Source: CAD feature listing. Evaluate the final solid. Frame: model axes, mm. A direction names the side the tool comes from. Coordinates: 2 decimals unless noted, no trailing zeros. Write each loop counter-clockwise with the first axis right and the second up, starting at its lowest first coordinate (ties: lowest second). Pieces come first, ordered by that corner, then holes. Notation, with made-up numbers: (86, -26.5) - (137, -26.5) arc R9 ccw to (137, -14.5) - close; hole circle Ø5 at (-13.75, -36). An arc over 180 degrees is marked (long way). One line per question, with ' | ' between items. Start each with the question number.
Q1. Draft query along Y for faces 1 (the face through (15, -9, 2)), 2 (the face through (-1.301, 19.143, 2.958)), 3 (the face through (14.43, -26.6, 7.04)), 4 (the face through (-12.341, -18.443, 6.958)). Return one class per face: +Y half, -Y half, draft (parallel to the pull), parting line (faces both ways), or undercut.
Q2. Contact query for flat-ended pins moving along their axis: P1, Ø1, axis at x = 11, y = -10, coming from the +Z side; P2, Ø17.5, axis at x = 2, y = 23.5, coming from the +Z side; P3, Ø3, axis at x = 2.5, z = 6, coming from the +Y side. Output: stop coordinate, or through.
Q3. Cut plane A-A, the plane y = 25. Return loops of the section in (x, z).
Q4. Access query for faces 5 (the face through (2, -26, 7)), 6 (the face through (-1.041, 32.932, 4.986)), 7 (the face through (11.43, -17.72, -3.04)). Directions: +Z, -Z, +X, -X, +Y, -Y. A direction counts if a zero-diameter tool reaches every point of the face in a straight line with its end or side. Return the directions, or none.
Q5. Cut plane B-B, the plane y = -10. Return loops of the section in (x, z), plus the area to 3 significant figures.
Q6. Line query: line 1 (Z direction, x = 5, y = 10); line 2 (X direction, y = 19.5, z = 3.25); line 3 (Y direction, x = 0, z = 1.85). Output: solid intervals per line, ascending.
```python
from build123d import *

# Parameters (mm, degrees)
F1_DEPTH = 10
F0_R     = 8
F2_DEPTH = 4
F0_R_2   = 6
F3_DEPTH = 6
F5_R     = 2
F7_DEPTH = 6
F8_R     = 1.5


with BuildPart() as f1:
    # F0 (on Top) → F1 (new body)
    with BuildSketch(Plane.XY):
        with BuildLine():
            Line((15, -37.5), (15, -26))
            Line((15, -26), (-9.9611850455, -26))
            add(Edge.make_bspline(
                [(-11.8869803846, -23.3454480823), (-11.8503261617, -24.0200703773), (-11.7257091732, -24.4668508278), (-11.1064253641, -25.4653853658), (-10.3231083129, -25.9576724499), (-9.9611850455, -26)],
                knots=[0, 0, 0, 0, 0.3405412191, 0.6578755277, 1, 1, 1, 1], degree=3))
            Line((-11.8869803846, -23.3454480823), (-11.8869803846, -21))
            ThreePointArc((-11.8869803846, -21), (-12.3717296786, -18.4168176701), (-15, -18.4196364135))
            Line((-15, -18.4196364135), (-15, -26))
            add(Edge.make_bspline(
                [(-15, -26), (-10.2944150567, -32.0423617959), (3.415344283, -37.3965017498), (15, -37.5)],
                knots=[0, 0, 0, 0, 32.1286476528, 32.1286476528, 32.1286476528, 32.1286476528], degree=3))
        make_face()
    extrude(amount=F1_DEPTH)


with BuildPart() as f2:
    # F0 (on Top) → F2 (new body)
    with BuildSketch(Plane.XY):
        with BuildLine():
            ThreePointArc((15, 32.5), (13.5355339059, 36.0355339059), (10, 37.5))
            Line((10, 37.5), (-10, 37.5))
            ThreePointArc((-10, 37.5), (-13.5355339059, 36.0355339059), (-15, 32.5))
            Line((-15, 32.5), (-15, -18.4196364135))
            ThreePointArc((-15, -18.4196364135), (-12.3717296786, -18.4168176701), (-11.8869803846, -21))
            Line((-11.8869803846, -21), (-11.8869803846, -23.3454480823))
            add(Edge.make_bspline(
                [(-11.8869803846, -23.3454480823), (-11.8503261617, -24.0200703773), (-11.7257091732, -24.4668508278), (-11.1064253641, -25.4653853658), (-10.3231083129, -25.9576724499), (-9.9611850455, -26)],
                knots=[0, 0, 0, 0, 0.3405412191, 0.6578755277, 1, 1, 1, 1], degree=3))
            Line((-9.9611850455, -26), (15, -26))
            Line((15, -26), (15, 32.5))
        make_face()
        with Locations((0, 25)):
            Circle(F0_R, mode=Mode.SUBTRACT)
    extrude(amount=F2_DEPTH)

    # F0 (on Top) → F3 (join)
    with BuildSketch(Plane.XY):
        with Locations((0, 25)):
            Circle(F0_R)
        with Locations((0, 25)):
            Circle(F0_R_2, mode=Mode.SUBTRACT)
    extrude(amount=F3_DEPTH)

    # F4: union F1
    add(f1.part)

    # F5
    f5_edges = [f2.edges().sort_by_distance(p)[0] for p in [
        (15, -26, 7),
        (15, -37.5, 5),
    ]]
    fillet(f5_edges, radius=F5_R)

    # F6 (on face) → F7 (join)
    with BuildSketch(Plane(origin=(0, 0, 0), x_dir=(1, 0, 0), z_dir=(0, 0, -1))):
        with BuildLine():
            add(Edge.make_bspline(
                [(11, 37.2695901222), (11.6289216889, 37.3346734853), (12.2554361711, 37.3865849072), (12.8779100925, 37.4246547986)],
                knots=[28.4914152983, 28.4914152983, 28.4914152983, 28.4914152983, 30.1861311863, 30.1861311863, 30.1861311863, 30.1861311863], degree=3))
            Line((11, 37.2695901222), (11, 17.2695901222))
            Line((11, 17.2695901222), (15, 17.2695901222))
            Line((15, 17.2695901222), (15, 35.4283847632))
            add(Edge.make_bspline(
                [(12.8779100925, 37.4246547986), (12.9997851475, 37.4321085568), (13.1257670983, 37.4308511004), (13.2548827191, 37.4198425025), (13.3858269049, 37.3981737159), (13.516965577, 37.3652625635), (13.7771948673, 37.2763649582), (13.9062664101, 37.2201858037), (14.0319471175, 37.1523455077), (14.1523190287, 37.0732018707), (14.2655986066, 36.9836823621), (14.4751385881, 36.7865661207), (14.571406291, 36.6789625216), (14.6577504243, 36.5636464215), (14.7331363723, 36.4423414141), (14.7970899201, 36.3169400414), (14.9017074178, 36.0626228243), (14.9425625457, 35.9337377832), (14.9721844022, 35.8043605761), (14.9910543263, 35.676157773), (15, 35.5504875377), (15, 35.4283847632)],
                knots=[0, 0, 0, 0, 0, 0, 0, 0.2489631265, 0.2489631265, 0.2489631265, 0.2489631265, 0.2489631265, 0.5, 0.5, 0.5, 0.5, 0.5, 0.7510368735, 0.7510368735, 0.7510368735, 0.7510368735, 0.7510368735, 1, 1, 1, 1, 1, 1, 1], degree=6))
        make_face()
    extrude(amount=F7_DEPTH)

    # F8
    f8_edges = [f2.edges().sort_by_distance(p)[0] for p in [
        (11, -17.26959, -3),
        (15, -17.26959, -3),
        (11, -37.26959, -3),
    ]]
    fillet(f8_edges, radius=F8_R)


solid = f2.part
```
Reply:
1) face 1: draft | face 2: undercut | face 3: +Y half | face 4: undercut
2) P1: stops at z = 4 | P2: stops at z = 6 | P3: stops at y = 32.94
3) outline: (-15, 0) - (-6, 0) - (-6, 6) - (-8, 6) - (-8, 4) - (-15, 4) - close; (6, 0) - (15, 0) - (15, 4) - (8, 4) - (8, 6) - (6, 6) - close
4) face 5: +Z, +X | face 6: +Z | face 7: -Z, -X, +Y
5) outline: (-15, 0) - (15, 0) - (15, 4) - (-15, 4) - close | area: 120 mm^2
6) line 1: z = 0 to 4 | line 2: x = -15 to -2.4, 2.4 to 15 | line 3: y = -34.9 to 19, 31 to 37.5
